```python
from build123d import *

# Parameters (mm, degrees)
SKETCH2_R          = 2.0193
CUT_EXTRUDE1_DEPTH = 25


with BuildPart() as part:
    # Sketch1 → Revolve1 (revolve)
    with BuildSketch(Plane(origin=(0, 0, 0), x_dir=(0, 0, -1), z_dir=(1, 0, 0)), mode=Mode.PRIVATE) as revolve1_sk:
        Polygon((185, 0), (185, 7), (35, 7), (35, 6), (-7.5, 6), (-7.5, 0), align=None)
    revolve(revolve1_sk.sketch.rotate(Axis((0, 0, 0), (0, 0, -1)), 90), axis=Axis((0, 0, 0), (0, 0, -1)))

    # Sketch2 → Cut-Extrude1 (cut)
    with BuildSketch(Plane.XY.offset(7.5)):
        Circle(SKETCH2_R)
    extrude(amount=-CUT_EXTRUDE1_DEPTH, mode=Mode.SUBTRACT)


solid = part.part
```
Check sheet for the modelled part. Datum: model origin and axes. Units: mm. A direction names the side the tool comes from. Round coordinates to 2 decimals unless told otherwise and drop trailing zeros. Order: outer loops, then holes, each group sorted by start corner. A loop starts at its lowest first (then second) coordinate and runs counter-clockwise, first axis right, second up.
1) Section check A-A (y = 0). Record the boundary of the cut face in (x, z).
2) Section check C-C (z = -152). Record the boundary of the cut face in (x, y), and give its area (3 significant figures).
3) Go/stop test with flat-tipped pins: pin 1 Ø1.5 at (x, z) = (4, -116) entering from +Y; pin 2 Ø3 at (y, z) = (-3.5, -140) entering from +X. Record where each tip stops, or that it passes through.
4) Mould release check, pull along X, two halves, no side actions. Record for faces 3 (the flat face through (3, 0, 7.5)), 4 (the cylindrical face through (1.926, 0.607, -4.825)), 5 (the flat face through (0, 0, -17.5)), 6 (the cylindrical face through (5.723, -1.802, -13.452)): +X half, -X half, draft (parallel to the pull), parting line (faces both ways), or undercut.
5) Scan lines: line 1 (Y direction, x = 0, z = -10.25); line 2 (X direction, y = -0.25, z = -158.5); line 3 (Z direction, x = 1, y = -0.5). Record each from-to range of solid material in increasing order.
6) Tool access check on faces 1 (the flat face through (0, 0, -185)), 2 (the flat face through (6, -2, -35)). Record the directions out of +Z, -Z, +X, -X, +Y, -Y that give a thin tool (end or side, any length) a straight path to the whole face; none if there is none.
7) Section check D-D (z = -25). Record the boundary of the cut face in (x, y), and give its area (3 significant figures).
Result:
1. outline: (-7, -185) - (7, -185) - (7, -35) - (6, -35) - (6, 7.5) - (2.02, 7.5) - (2.02, -17.5) - (-2.02, -17.5) - (-2.02, 7.5) - (-6, 7.5) - (-6, -35) - (-7, -35) - close
2. outline: circle Ø14 at (0, 0)
2. area: 154 mm2
3. pin 1: stops at y = 6.2
3. pin 2: stops at x = 6.71
4. face 3: draft
4. face 4: undercut
4. face 5: undercut
4. face 6: parting line
5. line 1: y = -6 to -2.02, 2.02 to 6
5. line 2: x = -7 to 7
5. line 3: z = -185 to -17.5
6. face 1: -Z, +X, -X, +Y, -Y
6. face 2: +Z
7. outline: circle Ø12 at (0, 0)
7. area: 113 mm2
